Verification items for the finished model (mm, model axes). Face numbers are marked on the shaded views. A direction names the side the tool comes from. Round coordinates to 2 decimals unless told otherwise and drop trailing zeros. Write each loop counter-clockwise with the first axis right and the second up, starting at its lowest first coordinate (ties: lowest second). Pieces come first, ordered by that corner, then holes.
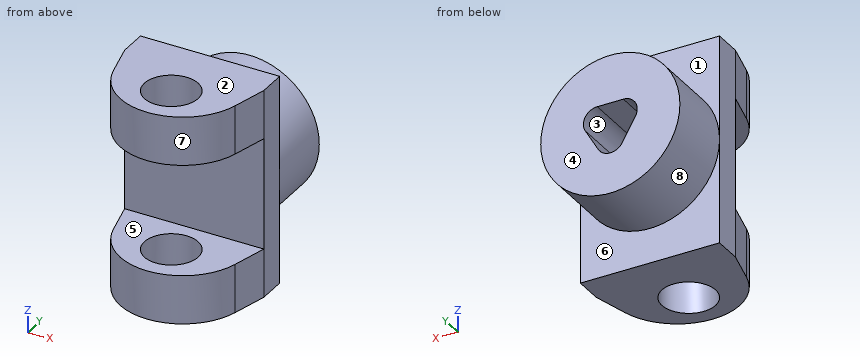
from build123d import *

# Parameters (mm, degrees)
SKETCH1_R               = 6.35
BOSS_EXTRUDE1_DEPTH     = 6.35
SKETCH1_5_W             = 12.7
SKETCH1_5_H             = 19.05
BOSS_EXTRUDE3_DEPTH     = 10.16
CUT_EXTRUDE1_DEPTH      = 7.62
CUT_EXTRUDE3_DEPTH      = 1
CUT_EXTRUDE3_DEPTH_BACK = 20.05
SKETCH5_4_R             = 2.4500078
CUT_EXTRUDE4_DEPTH      = 20.05
SKETCH6_W               = 10.16
SKETCH6_H               = 12.113180789
CUT_EXTRUDE5_DEPTH      = 7.35
CUT_EXTRUDE5_DEPTH_BACK = 7.35


with BuildPart() as part:
    # Sketch1 → Boss-Extrude1 (new body)
    with BuildSketch(Plane(origin=(0, 0, 0), x_dir=(1, 0, 0), z_dir=(0, 1, 0))):
        Circle(SKETCH1_R)
    extrude(amount=BOSS_EXTRUDE1_DEPTH)

    # Sketch1<5> → Boss-Extrude3 (add)
    with BuildSketch(Plane(origin=(0, 0, 0), x_dir=(1, 0, 0), z_dir=(0, 1, 0))):
        Rectangle(SKETCH1_5_W, SKETCH1_5_H)
    extrude(amount=-BOSS_EXTRUDE3_DEPTH)

    # Sketch3 → Cut-Extrude1 (cut)
    with BuildSketch(Plane(origin=(0, 6.35, 0), x_dir=(1, 0, 0), z_dir=(0, 1, 0))):
        with BuildLine():
            Line((-1.099852263, 2.007933515), (-2.288847564, -0.051466757))
            ThreePointArc((-2.288847564, -0.051466757), (-2.288847564, -1.321466757), (-1.188995301, -1.956466757))
            Line((-1.188995301, -1.956466757), (1.188995301, -1.956466757))
            ThreePointArc((1.188995301, -1.956466757), (2.288847564, -1.321466757), (2.288847564, -0.051466757))
            Line((2.288847564, -0.051466757), (1.099852263, 2.007933515))
            ThreePointArc((1.099852263, 2.007933515), (0, 2.642933515), (-1.099852263, 2.007933515))
        make_face()
    extrude(amount=-CUT_EXTRUDE1_DEPTH, mode=Mode.SUBTRACT)

    # Sketch5 → Cut-Extrude3 (cut, two sides)
    with BuildSketch(Plane(origin=(0, 0, -9.525), x_dir=(-1, 0, 0), z_dir=(0, 0, -1))) as cut_extrude3_sk:
        with BuildLine():
            Line((6.35, -2.54), (5.551173901, -5.743916488))
            ThreePointArc((5.551173901, -5.743916488), (0, -10.080968867), (-5.551173901, -5.743916488))
            Line((-5.551173901, -5.743916488), (-6.35, -2.54))
            Line((-6.35, -2.54), (-6.35, -10.16))
            Line((-6.35, -10.16), (6.35, -10.16))
            Line((6.35, -10.16), (6.35, -2.54))
        make_face()
    extrude(amount=CUT_EXTRUDE3_DEPTH, mode=Mode.SUBTRACT)
    extrude(cut_extrude3_sk.sketch, amount=-CUT_EXTRUDE3_DEPTH_BACK, mode=Mode.SUBTRACT)

    # Sketch5<4> → Cut-Extrude4 (cut, through all)
    with BuildSketch(Plane(origin=(0, 0, -9.525), x_dir=(-1, 0, 0), z_dir=(0, 0, -1))):
        with Locations((0, -6.219754937)):
            Circle(SKETCH5_4_R)
    extrude(amount=-CUT_EXTRUDE4_DEPTH, mode=Mode.SUBTRACT)

    # Sketch6 → Cut-Extrude5 (cut, two sides)
    with BuildSketch(Plane(origin=(0, 0, 0), x_dir=(0, 0, -1), z_dir=(1, 0, 0))) as cut_extrude5_sk:
        with Locations((0, -8.596590394)):
            Rectangle(SKETCH6_W, SKETCH6_H)
    extrude(amount=CUT_EXTRUDE5_DEPTH, mode=Mode.SUBTRACT)
    extrude(cut_extrude5_sk.sketch, amount=-CUT_EXTRUDE5_DEPTH_BACK, mode=Mode.SUBTRACT)


solid = part.part
Q1. Tool access check on the marked faces 4, 5, 6, 7 and 8. Record the directions out of +Z, -Z, +X, -X, +Y, -Y that give a thin tool (end or side, any length) a straight path to the whole face; none if there is none.
Recorded:
face 4: +Z, -Z, +X, -X, +Y
face 5: +X, -X, -Y
face 6: -Z, +Y
face 7: +Z, -Z, -Y
face 8: +Y
Q2. Material ranges on line 1 along Y through (x, z) = (0, -7.9); line 2 along Z through (x, y) = (3.25, -8.5) (3 decimals); line 3 along Y through (x, z) = (-2.25, -1), recorded low to high.
Recorded:
line 1: y = -10.08 to -8.67, -3.77 to 0
line 2: z = -9.525 to -5.08, 5.08 to 9.525
line 3: y = -2.54 to 6.35
Q3. Sectioned sample at B-B (y = -4.75). Enter the section's corners in (x, z) (3 decimals), plus the area to 3 significant figures.
Recorded:
outline: (-5.799, -9.525) - (-1.96, -9.525) - (-1.96, -5.08) - (-5.799, -5.08) - close; (-5.799, 5.08) - (-1.96, 5.08) - (-1.96, 9.525) - (-5.799, 9.525) - close; (1.96, -9.525) - (5.799, -9.525) - (5.799, -5.08) - (1.96, -5.08) - close; (1.96, 5.08) - (5.799, 5.08) - (5.799, 9.525) - (1.96, 9.525) - close
area: 68.3 mm2
Q4. Sectioned sample at A-A (x = 0). Enter the section's corners in (y, z) (3 decimals).
Recorded:
outline: (-10.081, -9.525) - (-8.67, -9.525) - (-8.67, -5.08) - (-10.081, -5.08) - close; (-10.081, 5.08) - (-8.67, 5.08) - (-8.67, 9.525) - (-10.081, 9.525) - close; (-3.77, -9.525) - (0, -9.525) - (0, -6.35) - (6.35, -6.35) - (6.35, -2.643) - (-1.27, -2.643) - (-1.27, 1.956) - (6.35, 1.956) - (6.35, 6.35) - (0, 6.35) - (0, 9.525) - (-3.77, 9.525) - (-3.77, 5.08) - (-2.54, 5.08) - (-2.54, -5.08) - (-3.77, -5.08) - close
Q5. Release check for a two-part mould opening along Z. For the marked faces 1, 2 and 3 record: released by +Z, released by -Z, zero draft, split by the parting line, or undercut.
Recorded:
face 1: zero draft
face 2: released by +Z
face 3: undercut
Q6. Depth check by flat-ended pin: P1, Ø4, axis at x = -2.5, z = -2, coming from the -Y side; P2, Ø5, axis at x = 2.5, y = 3, coming from the -Z side; P3, Ø1, axis at x = -0.5, y = -7, coming from the -Z side; P4, Ø1, axis at x = -4, z = -5.5, coming from the -Y side. Enter the tip coordinate at first touch or a pass-through.
Recorded:
P1: stops at y = -2.54
P2: stops at z = -6.35
P3: passes through
P4: stops at y = -8.89
Q7. Sectioned sample at C-C (y = -0.75). Enter the section's corners in (x, z) (3 decimals), plus the area to 3 significant figures.
Recorded:
outline: (-6.35, -9.525) - (6.35, -9.525) - (6.35, 9.525) - (-6.35, 9.525) - close; hole (-2.289, 0.051) - (-1.1, -2.008) arc R1.27 ccw to (1.1, -2.008) - (2.289, 0.051) arc R1.27 ccw to (1.189, 1.956) - (-1.189, 1.956) arc R1.27 ccw to start
area: 225 mm2
